Input: dimensioned drawing with shaded views. Units: mm. Origin: part minimum x, y, z. A direction names the side the tool comes from. Coordinates: 2 decimals unless noted, no trailing zeros. Loops run counter-clockwise (first coordinate to the right, second up) from the corner with the lowest first, then second, coordinate; pieces in that order, holes last.
(1) Set-up query: the marked faces 1, 2 and 3. Return all of +Z, -Z, +X, -X, +Y, -Y with unobstructed straight access to the full face (end or side cutting, diameter ignored); none if empty.
(2) Contact query for flat-ended pins moving along their axis: P1, Ø3.5, axis at x = 20.5, z = 44, coming from the +Y side; P2, Ø2, axis at x = 30, z = 45.5, coming from the +Y side; P3, Ø11.5, axis at x = 27, y = 12.5, coming from the +Z side; P4, Ø10, axis at y = 22, z = 17.5, coming from the -X side. Output: stop coordinate, or through.
(3) Section A-A, the plane x = 30.5. Return loops of the section in (y, z), then the cut area to 3 significant figures.
(4) Section D-D, the plane x = 37. Return loops of the section in (y, z), then the cut area to 3 significant figures.
(5) Section B-B, the plane z = 9.5. Return loops of the section in (x, y), then the cut area to 4 significant figures.
(6) Section C-C, the plane y = 16.25. Return loops of the section in (x, z), then the cut area to 3 significant figures.
(7) Line query: L1, parallel to X at y = 0.7, z = 44; L2, parallel to Z at x = 7.5, y = 23.75; L3, parallel to Y at x = 34, z = 11.5. Output: solid intervals per line, ascending.
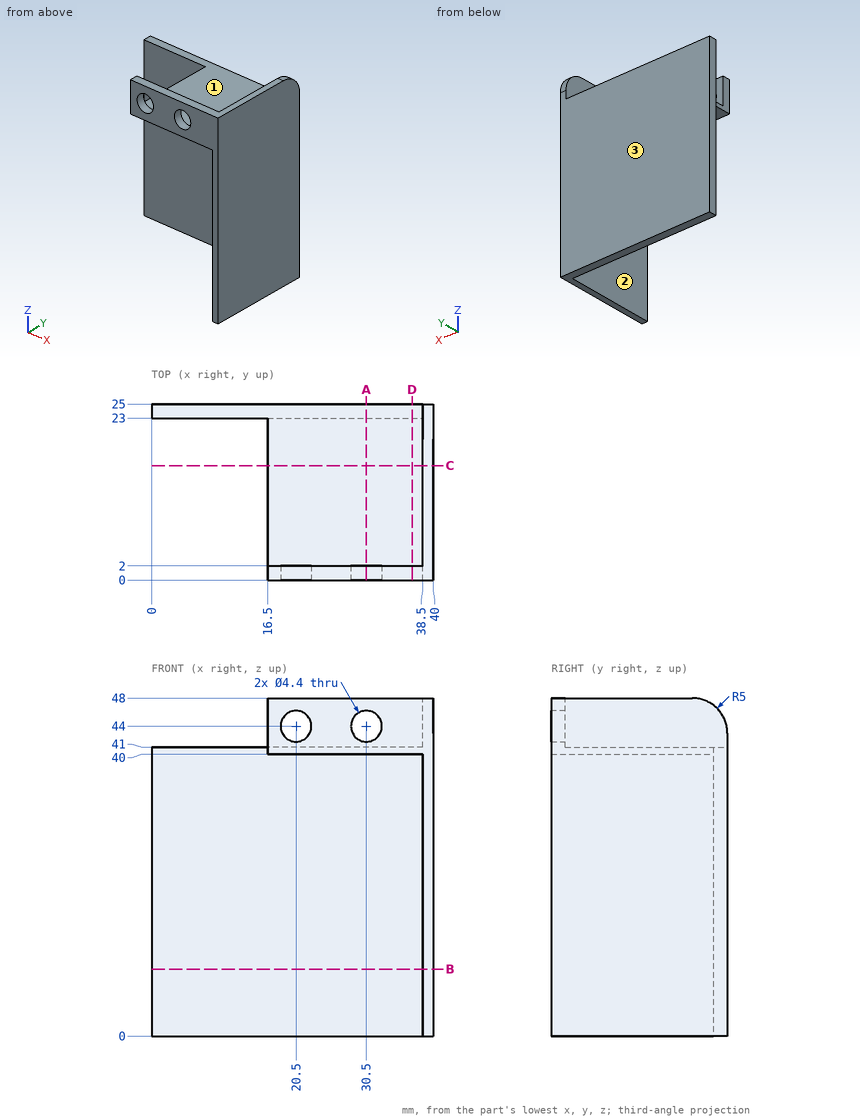
Report:
1. face 1: +Z, -X, +Y
1. face 2: -Z, -X, -Y
1. face 3: +Z, -Z, +X, -X, +Y
2. P1: passes through
2. P2: stops at y = 2
2. P3: stops at z = 41
2. P4: stops at x = 0
3. outline: (0, 40) - (23, 40) - (23, 0) - (25, 0) - (25, 41) - (2, 41) - (2, 41.8) - (0, 41.8) - close; (0, 46.2) - (2, 46.2) - (2, 48) - (0, 48) - close
3. area: 110 mm2
4. outline: (0, 40) - (23, 40) - (23, 0) - (25, 0) - (25, 41) - (2, 41) - (2, 48) - (0, 48) - close
4. area: 119 mm2
5. outline: (0, 23) - (38.5, 23) - (38.5, 0) - (40, 0) - (40, 25) - (0, 25) - close
5. area: 114.5 mm2
6. outline: (16.5, 40) - (38.5, 40) - (38.5, 0) - (40, 0) - (40, 48) - (38.5, 48) - (38.5, 41) - (16.5, 41) - close
6. area: 94.0 mm2
7. L1: x = 16.5 to 18.3, 22.7 to 28.3, 32.7 to 40
7. L2: z = 0 to 41
7. L3: y = 23 to 25
